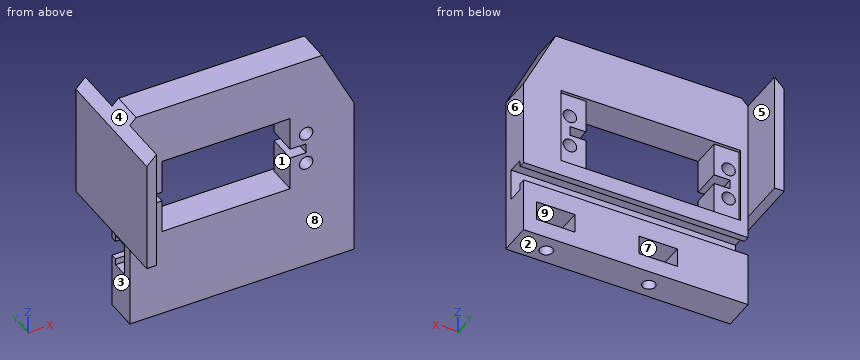
from build123d import *

# Parameters (mm, degrees)
SKETCH_1_W           = 80
SKETCH_1_H           = 60
SKETCH_1_R           = 2.1
SKETCH_1_W_2         = 40
SKETCH_1_H_2         = 24
EXTRUDE_1_DEPTH      = 10
CUT_EXTRUDE_1_DEPTH  = 80
SKETCH_5_W           = 5
SKETCH_5_H           = 3
CUT_EXTRUDE_2_DEPTH  = 80
SKETCH_7_W           = 56
SKETCH_7_H           = 24
CUT_EXTRUDE_3_DEPTH  = 1
SKETCH_8_W           = 40
SKETCH_8_H           = 40
EXTRUDE_2_DEPTH      = 3
SKETCH_9_W           = 10
SKETCH_9_H           = 60
CUT_EXTRUDE_4_DEPTH  = 10
CUT_EXTRUDE_11_DEPTH = 28
CUT_EXTRUDE_12_DEPTH = 28
SKETCH_24_W          = 10
SKETCH_24_H          = 10
EXTRUDE_3_DEPTH      = 70
SKETCH_25_W          = 12
SKETCH_25_H          = 6
CUT_EXTRUDE_13_DEPTH = 9
SKETCH_26_R          = 2
CUT_EXTRUDE_14_DEPTH = 8
CUT_EXTRUDE_15_REACH = 65.828


with BuildPart() as part:
    # 草圖1 → 填料-伸長1 (new body)
    with BuildSketch(Plane(origin=(0, 0, 0), x_dir=(1, 0, 0), z_dir=(0, 1, 0))):
        Rectangle(SKETCH_1_W, SKETCH_1_H)
        with Locations(Location((-34.5, -5, 0), (0, 0, 270))):
            Circle(SKETCH_1_R, mode=Mode.SUBTRACT)
        with Locations(Location((-34.5, 5, 0), (0, 0, 270))):
            Circle(SKETCH_1_R, mode=Mode.SUBTRACT)
        with Locations(Location((15, -5, 0), (0, 0, 270))):
            Circle(SKETCH_1_R, mode=Mode.SUBTRACT)
        with Locations(Location((15, 5, 0), (0, 0, 270))):
            Circle(SKETCH_1_R, mode=Mode.SUBTRACT)
        with Locations((-10, 0)):
            Rectangle(SKETCH_1_W_2, SKETCH_1_H_2, mode=Mode.SUBTRACT)
    extrude(amount=EXTRUDE_1_DEPTH)

    # 草圖4 → 除料-伸長1 (cut)
    with BuildSketch(Plane(origin=(40, 0, 0), x_dir=(0, 0, -1), z_dir=(1, 0, 0))):
        Polygon((17, 10), (17, 8), (15, 8), (15, 3), (25, 3), (25, 8), (23, 8), (23, 10), align=None)
    extrude(amount=-CUT_EXTRUDE_1_DEPTH, mode=Mode.SUBTRACT)

    # 草圖5 → 除料-伸長2 (cut)
    with BuildSketch(Plane(origin=(0, 10, 0), x_dir=(1, 0, 0), z_dir=(0, 1, 0))):
        with Locations((12.5, 0)):
            Rectangle(SKETCH_5_W, SKETCH_5_H)
        with Locations((-32.5, 0)):
            Rectangle(SKETCH_5_W, SKETCH_5_H)
    extrude(amount=-CUT_EXTRUDE_2_DEPTH, mode=Mode.SUBTRACT)

    # 草圖7 → 除料-伸長3 (cut)
    with BuildSketch(Plane(origin=(0, 10, 0), x_dir=(1, 0, 0), z_dir=(0, 1, 0))):
        with Locations((-9.7, 0)):
            Rectangle(SKETCH_7_W, SKETCH_7_H)
    extrude(amount=-CUT_EXTRUDE_3_DEPTH, mode=Mode.SUBTRACT)

    # 草圖8 → 填料-伸長2 (add)
    with BuildSketch(Plane.ZY.offset(40)):
        with Locations((10, 5)):
            Rectangle(SKETCH_8_W, SKETCH_8_H)
    extrude(amount=EXTRUDE_2_DEPTH)

    # 草圖9 → 除料-伸長4 (cut)
    with BuildSketch(Plane(origin=(0, 10, 0), x_dir=(1, 0, 0), z_dir=(0, 1, 0))):
        with Locations((35, 0)):
            Rectangle(SKETCH_9_W, SKETCH_9_H)
    extrude(amount=-CUT_EXTRUDE_4_DEPTH, mode=Mode.SUBTRACT)

    # 草圖22 → 除料-伸長11 (cut)
    with BuildSketch(Plane(origin=(0, 10, 0), x_dir=(1, 0, 0), z_dir=(0, 1, 0))):
        Polygon((-43, -25), (-43, -30), (-38, -30), align=None)
    extrude(amount=-CUT_EXTRUDE_11_DEPTH, mode=Mode.SUBTRACT)

    # 草圖23 → 除料-伸長12 (cut)
    with BuildSketch(Plane(origin=(0, 25, 0), x_dir=(1, 0, 0), z_dir=(0, 1, 0))):
        Polygon((-43, -30), (-38, -30), (-43, -25), align=None)
    extrude(amount=-CUT_EXTRUDE_12_DEPTH, mode=Mode.SUBTRACT)

    # 草圖24 → 填料-伸長3 (add)
    with BuildSketch(Plane.ZY.offset(40)):
        with Locations((-35, 5)):
            Rectangle(SKETCH_24_W, SKETCH_24_H)
    extrude(amount=-EXTRUDE_3_DEPTH)

    # 草圖25 → 除料-伸長13 (cut)
    with BuildSketch(Plane(origin=(0, 10, 0), x_dir=(1, 0, 0), z_dir=(0, 1, 0))):
        with Locations((-12, 32)):
            Rectangle(SKETCH_25_W, SKETCH_25_H)
        with Locations((20, 32)):
            Rectangle(SKETCH_25_W, SKETCH_25_H)
    extrude(amount=-CUT_EXTRUDE_13_DEPTH, mode=Mode.SUBTRACT)

    # 草圖26 → 除料-伸長14 (cut)
    with BuildSketch(Plane(origin=(0, 0, -40), x_dir=(-1, 0, 0), z_dir=(0, 0, -1))):
        with Locations((-20, 4.723394197)):
            Circle(SKETCH_26_R)
        with Locations((12, 4.723394197)):
            Circle(SKETCH_26_R)
    extrude(amount=-CUT_EXTRUDE_14_DEPTH, mode=Mode.SUBTRACT)

    # 草圖27 → 除料-伸長15 (cut, up to next)
    with BuildSketch(Plane(origin=(0, 10, 0), x_dir=(1, 0, 0), z_dir=(0, 1, 0)), mode=Mode.PRIVATE) as cut_extrude_15_sk1:
        Polygon((30, -10), (20, -30), (30, -30), align=None)
    cut_extrude_15_tool1 = extrude(cut_extrude_15_sk1.sketch, amount=-CUT_EXTRUDE_15_REACH, mode=Mode.PRIVATE) & part.part
    add(cut_extrude_15_tool1.solids().sort_by_distance((26.666667, 10, 23.333333))[0], mode=Mode.SUBTRACT)


solid = part.part
Work out the finished part from the listing and answer in its coordinate system (mm). Face numbers are marked on the shaded views. A direction names the side the tool comes from. Coordinates: 2 decimals unless noted, no trailing zeros. Order: outer loops, then holes, each group sorted by start corner. A loop starts at its lowest first (then second) coordinate and runs counter-clockwise, first axis right, second up. Notation, with made-up numbers: (46, -7.75) - (63, -7.75) arc R24 cw to (63, 29.25) - close; hole circle Ø9 at (-4.5, 42.5). An arc over 180 degrees is marked (long way). Put each result on its own line as item: value. Start each with the question number.
1) Find section C-C (z = 18.5). Give the vertices of the cut face in (x, y).
2) Flat-ended cylindrical pins translate along their axes: pin 1 (6.5 mm diameter, centred on x = 15, z = -5, fed in from -Y); pin 2 (3.5 mm diameter, centred on x = -41.5, y = 7.5, fed in from -Z); pin 3 (4 mm diameter, centred on x = 16, z = 2, fed in from +Y); pin 4 (1.8 mm diameter, centred on x = 21.5, z = -30.5, fed in from +Y). Find the tip coordinate at first contact, or state that the pin passes through.
3) Find the intervals of material crossed by line 1 (X direction, y = 4, z = 5); line 2 (X direction, y = 3, z = 0.5); line 3 (X direction, y = 7.5, z = -4), in increasing order. Write a range as from..to.
4) Find section B-B (x = -16.5). Give the vertices of the cut face in (y, z), plus the area to 3 significant figures.
5) Find section D-D (x = -5). Give the vertices of the cut face in (y, z), plus the area to 3 significant figures.
6) For a pull along X with two mould halves and no side action, classify the marked faces 6, 7, 8 and 9 as released by +X, released by -X, zero draft, split by the parting line, or undercut.
7) For the marked faces 1, 2, 3, 4 and 5, determine the directions among +Z, -Z, +X, -X, +Y, -Y from which every point of the face is accessible in a straight line to the end or side of a thin tool.
8) Find section A-A (z = -5). Give the vertices of the cut face in (x, y).
Results list:
1. outline: (-43, -15) - (-40, -15) - (-40, 0) - (25.75, 0) - (25.75, 10) - (-40, 10) - (-40, 25) - (-43, 25) - close
2. pin 1: stops at y = 0
2. pin 2: stops at z = -40
2. pin 3: stops at y = 9
2. pin 4: stops at y = 1
3. line 1: x = -43..-36.6, -32.4..-30, 10..12.9, 17.1..30
3. line 2: x = -43..-35, 15..30
3. line 3: x = -43..-36.35, -32.65..-30, 10..13.15, 16.85..30
4. outline: (0, -40) - (10, -40) - (10, -35) - (1, -35) - (1, -29) - (10, -29) - (10, -23) - (8, -23) - (8, -25) - (3, -25) - (3, -15) - (8, -15) - (8, -17) - (10, -17) - (10, -12) - (0, -12) - close; (0, 12) - (10, 12) - (10, 30) - (0, 30) - close
4. area: 344 mm^2
5. outline: (0, -40) - (10, -40) - (10, -23) - (8, -23) - (8, -25) - (3, -25) - (3, -15) - (8, -15) - (8, -17) - (10, -17) - (10, -12) - (0, -12) - close; (0, 12) - (10, 12) - (10, 30) - (0, 30) - close
5. area: 398 mm^2
6. face 6: released by +X
6. face 7: undercut
6. face 8: zero draft
6. face 9: undercut
7. face 1: +Y, -Y
7. face 2: -Z, +X, -X, +Y, -Y
7. face 3: -Z, -X, +Y, -Y
7. face 4: +Z, -X, +Y, -Y
7. face 5: +Z, -Z, +X, +Y
8. outline: (-43, -15) - (-40, -15) - (-40, 0) - (-36.6, 0) - (-36.6, 9) - (-37.7, 9) - (-37.7, 10) - (-40, 10) - (-40, 25) - (-43, 25) - close; (-32.4, 0) - (-30, 0) - (-30, 9) - (-32.4, 9) - close; (10, 0) - (12.9, 0) - (12.9, 9) - (10, 9) - close; (17.1, 0) - (30, 0) - (30, 10) - (18.3, 10) - (18.3, 9) - (17.1, 9) - close
